```python
from build123d import *

# Parameters (mm, degrees)
SKETCH1_R           = 5.5
SKETCH1_R_2         = 2
BOSS_EXTRUDE1_DEPTH = 2
SKETCH2_R           = 4.5
SKETCH2_R_2         = 4
SKETCH2_R_3         = 3
SKETCH2_R_4         = 2.75
CUT_EXTRUDE1_DEPTH  = 0.5
CUT_EXTRUDE2_START  = -0.5
SKETCH3_R           = 4.5
SKETCH3_R_2         = 4
SKETCH3_R_3         = 3
SKETCH3_R_4         = 2.75
CUT_EXTRUDE2_DEPTH  = 0.5
CHAMFER1_SIZE       = 0.3


with BuildPart() as part:
    # Sketch1 → Boss-Extrude1 (new body)
    with BuildSketch(Plane(origin=(0, 0, 0), x_dir=(1, 0, 0), z_dir=(0, 1, 0))):
        with Locations(Location((0, 0, 0), (0, 0, 270))):
            Circle(SKETCH1_R)
        with Locations(Location((0, 0, 0), (0, 0, 270))):
            Circle(SKETCH1_R_2, mode=Mode.SUBTRACT)
    extrude(amount=BOSS_EXTRUDE1_DEPTH)

    # Sketch2 → Cut-Extrude1 (cut)
    # profile 1 of 2: a face of its own
    with BuildSketch(Plane(origin=(0, 2, 0), x_dir=(1, 0, 0), z_dir=(0, 1, 0))):
        with Locations(Location((0, 0, 0), (0, 0, 270))):
            Circle(SKETCH2_R)
        with Locations(Location((0, 0, 0), (0, 0, 270))):
            Circle(SKETCH2_R_2, mode=Mode.SUBTRACT)
    # profile 2 of 2: a face of its own
    with BuildSketch(Plane(origin=(0, 2, 0), x_dir=(1, 0, 0), z_dir=(0, 1, 0))):
        with Locations(Location((0, 0, 0), (0, 0, 270))):
            Circle(SKETCH2_R_3)
        with Locations(Location((0, 0, 0), (0, 0, 270))):
            Circle(SKETCH2_R_4, mode=Mode.SUBTRACT)
    extrude(amount=-CUT_EXTRUDE1_DEPTH, mode=Mode.SUBTRACT)

    # Sketch3 → Cut-Extrude2 (cut)
    # profile 1 of 2: a face of its own
    with BuildSketch(Plane.XZ.offset(CUT_EXTRUDE2_START)):
        with Locations(Location((0, 0, 0), (0, 0, 90))):
            Circle(SKETCH3_R)
        with Locations(Location((0, 0, 0), (0, 0, 90))):
            Circle(SKETCH3_R_2, mode=Mode.SUBTRACT)
    # profile 2 of 2: a face of its own
    with BuildSketch(Plane.XZ.offset(CUT_EXTRUDE2_START)):
        with Locations(Location((0, 0, 0), (0, 0, 90))):
            Circle(SKETCH3_R_3)
        with Locations(Location((0, 0, 0), (0, 0, 90))):
            Circle(SKETCH3_R_4, mode=Mode.SUBTRACT)
    extrude(amount=CUT_EXTRUDE2_DEPTH, mode=Mode.SUBTRACT)

    # Chamfer1
    chamfer1_edges = [part.edges().sort_by_distance(p)[0] for p in [
        (0, 0, -5.5),
        (0, 2, -5.5),
    ]]
    chamfer(chamfer1_edges, length=CHAMFER1_SIZE)


solid = part.part
```
Geometry check sheet. Reference: the model listing, model coordinates, mm. A direction names the side the tool comes from. Give positions to 0.01 mm unless a question says otherwise; leave off trailing zeros. Use a Markdown table: item, result.
Q1. Draft check along Z on faces 4 (the face through (-2, 0, 1)), 5 (the face through (-3.905, 1.754, -0.867)), 6 (the face through (-5.37, 0.99, -1.19)). Enter one of: pulls with the +Z half, pulls with the -Z half, needs draft (parallel to the pull), parting line crosses it, or undercut.
Computed:
| item | result |
|---|---|
| face 4 | needs draft |
| face 5 | undercut |
| face 6 | parting line crosses it |
Q2. Go/stop test with flat-tipped pins: P1, Ø1, axis at x = 4, y = 0.5, coming from the -Z side; P2, Ø3.5, axis at x = 0, z = 0, coming from the -Y side. Record where each tip stops, or that it passes through.
Computed:
| item | result |
|---|---|
| P1 | stops at z = -4.24 |
| P2 | passes through |
Q3. Set-up check for faces 1 (the face through (-2.685, 1.754, -0.596)), 2 (the face through (-1.352, 0.254, 4.292)), 3 (the face through (-2, 1, 0)): record each of +Z, -Z, +X, -X, +Y, -Y from which the full face is reachable in a straight line by a thin tool's end or side.
Computed:
| item | result |
|---|---|
| face 1 | +Y |
| face 2 | -Y |
| face 3 | +Y, -Y |
Q4. Thickness scan on L1, parallel to X at y = 1.3, z = 0; L2, parallel to Y at x = -3.5, z = 2.75; L3, parallel to X at y = 0.25, z = 0. Record the ranges inside material, lowest first. Write a range as [from, to].
Computed:
| item | result |
|---|---|
| L1 | x = [-5.5, -2], [2, 5.5] |
| L2 | y = [0.5, 1.5] |
| L3 | x = [-5.45, -4.5], [-4, -3], [-2.75, -2], [2, 2.75], [3, 4], [4.5, 5.45] |
